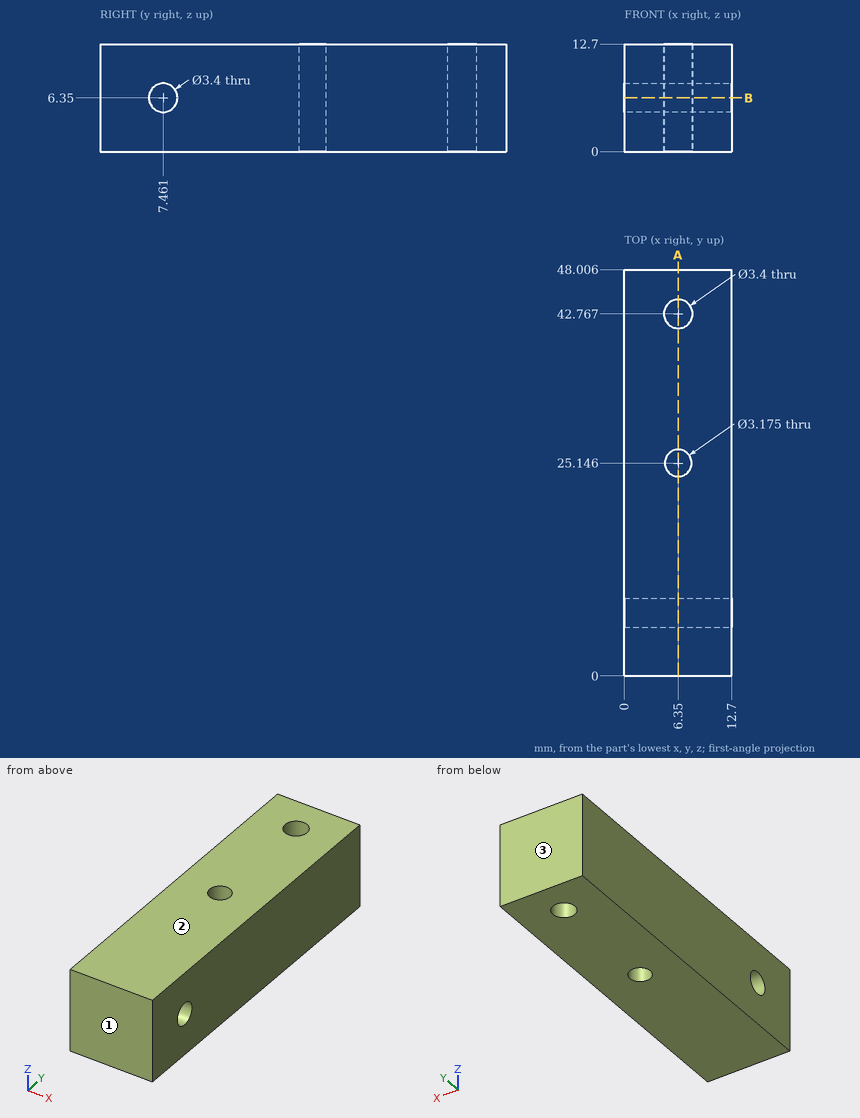
Verification items for this drawing (mm, ordinates from the low corner). Coordinates: 2 decimals unless noted, no trailing zeros. Loops run counter-clockwise (first coordinate to the right, second up) from the corner with the lowest first, then second, coordinate; pieces in that order, holes last. Notation, with made-up numbers: (1.25, 86) - (33.25, 86) arc R23 cw to (33.25, 94) - close; hole circle Ø7 at (-7, 23.25). An arc over 180 degrees is marked (long way). Use one line per item in the form item = value. Start each with the question number.
Item 1: Section check A-A, the plane x = 6.35. Enter the section's corners in (y, z), and give its area (3 significant figures).
Item 2: Mould release check, pull along Y, two halves, no side actions. Record for the marked faces 1, 2 and 3: +Y half, -Y half, draft (parallel to the pull), parting line (faces both ways), or undercut.
Item 3: Section check B-B, the plane z = 6.35. Give the number of separate pieces and of enclosed holes in the cut face.
Item 4: Thickness scan on probe 1 along Y at (x, z) = (6.5, 1) (1 decimal); probe 2 along Y at (x, z) = (12, 6.25); probe 3 along Y at (x, z) = (5.25, 6.5) (1 decimal). Record the ranges inside material, lowest first.
Computed:
q1.outline = (0, 0) - (23.56, 0) - (23.56, 12.7) - (0, 12.7) - close; (26.73, 0) - (41.07, 0) - (41.07, 12.7) - (26.73, 12.7) - close; (44.47, 0) - (48.01, 0) - (48.01, 12.7) - (44.47, 12.7) - close; hole circle Ø3.4 at (7.46, 6.35)
q1.area = 517 mm2
q2.face_1 = -Y half
q2.face_2 = draft
q2.face_3 = +Y half
q3.separate_pieces = 2
q3.enclosed_holes = 2
q4.probe_1 = 0 to 23.6, 26.7 to 41.1, 44.5 to 48
q4.probe_2 = 0 to 5.76, 9.16 to 48.01
q4.probe_3 = 0 to 5.8, 9.2 to 24, 26.3 to 41.5, 44.1 to 48
